Autodesk Inventor part; units mm, degrees
ref_plane "YZ Plane" through (0, 0, 0) normal (1, 0, 0) x (0, 1, 0)
ref_plane "XZ Plane" through (0, 0, 0) normal (0, 1, 0) x (-1, 0, 0)
ref_plane "XY Plane" through (0, 0, 0) normal (0, 0, 1) x (1, 0, 0)
sketch "Sketch9" plane through (0, 0, 0) normal (0, 1, 0) x (-1, 0, 0)
  line L0 (25, 25) -> (-25, 25)
  line L1 (-25, 25) -> (-25, -25)
  line L2 (-25, -25) -> (25, -25)
  line L3 (25, -25) -> (25, 25)
  line L4 (25, 25) -> (-25, -25) construction
  line L5 (-25, 25) -> (25, -25) construction
  line L6 (-23, 23) -> (23, 23)
  line L7 (23, 23) -> (23, -23)
  line L8 (23, -23) -> (-23, -23)
  line L9 (-23, -23) -> (-23, 23)
  point P0 (0, 0)
  dimension "d172" = 50
  dimension "d173" = 50
  dimension "d174" = 2
extrude "Extrusion3" add sketch "Sketch9" against normal blind 1350
sketch "Sketch10" plane through (0, 0, 0) normal (1, 0, 0) x (0, 1, 0)
  line L0 (0, 25) -> (0, -25) construction
  line L1 (0, 25) -> (-1350, 25) construction
  line L2 (-1350, -25) -> (-1350, 25) construction
  line L3 (0, -25) -> (-1350, -25) construction
  line L4 (-43.5, 8.5) -> (-26.5, 8.5)
  line L5 (-26.5, 8.5) -> (-26.5, -8.5)
  line L6 (-26.5, -8.5) -> (-43.5, -8.5)
  line L7 (-43.5, -8.5) -> (-43.5, 8.5)
  line L8 (-43.5, 8.5) -> (-26.5, -8.5) construction
  line L9 (-26.5, 8.5) -> (-43.5, -8.5) construction
  line L10 (0, 0) -> (50, 0)
  circle A0 centre (-35, 0) radius 8.5
  dimension "d177" = 17
  dimension "d178" = 17
  dimension "d181" = 50
  dimension "d190" = 35
extrude "Extrusion4" cut sketch "Sketch10" along normal through all contours A0
pattern_linear "Rectangular Pattern4" count 12 spacing 118 along (0, -1, 0) of "Extrusion4"
properties part number "TKS 3521 FDS way 1" material "Stainless Steel"
Geometry check sheet. Reference: the model listing, model coordinates, mm. A direction names the side the tool comes from. Coordinates: 2 decimals unless noted, no trailing zeros. Write each loop counter-clockwise with the first axis right and the second up, starting at its lowest first coordinate (ties: lowest second). Pieces come first, ordered by that corner, then holes. Notation, with made-up numbers: (65, -3.75) -> (102, -3.75) arc R6 ccw to (102, 7.25) -> close; hole circle Ø1 at (-25, 59). An arc over 180 degrees is marked (long way). One line per question, with ' | ' between items.
1. Depth check by flat-ended pin: pin 1 Ø13.5 at (y, z) = (-1097, 0) entering from +X. Enter the tip coordinate at first touch or a pass-through.
Answers:
pin 1: stops at x = -23
2. Set-up check for faces 1 (the flat face through (25, -666, 0)), 2 (the flat face through (0, -666, -23)): record each of +Z, -Z, +X, -X, +Y, -Y from which the full face is reachable in a straight line by a thin tool's end or side.
Answers:
face 1: +Z, -Z, +X, +Y, -Y | face 2: +Y, -Y
3. Draft check along Z on faces 3 (the flat face through (-25, -666, 0)), 4 (the flat face through (0, -666, 25)), 5 (the flat face through (23, -666, 0)). Enter one of: +Z half, -Z half, draft (parallel to the pull), parting line (faces both ways), or undercut.
Answers:
face 3: draft | face 4: +Z half | face 5: undercut
4. Thickness scan on probe 1 along X at (y, z) = (-1245.5, 11); probe 2 along Z at (x, y) = (24, -389). Record the ranges inside material, lowest first. Write a range as from..to.
Answers:
probe 1: x = -25..-23, 23..25 | probe 2: z = -25..-8.5, 8.5..25
5. Cross-section at B-B on y = -181. Record the cut outline in (x, z).
Answers:
outline: (-25, -25) -> (25, -25) -> (25, 25) -> (-25, 25) -> close; hole (-23, -23) -> (23, -23) -> (23, 23) -> (-23, 23) -> close
6. Cross-section at A-A on x = 1.5. Record the cut outline in (y, z).
Answers:
outline: (-1350, -25) -> (0, -25) -> (0, -23) -> (-1350, -23) -> close; (-1350, 23) -> (0, 23) -> (0, 25) -> (-1350, 25) -> close
